from build123d import *

# Parameters (mm, degrees)
EXTRUDE1_DEPTH     = 0.65
CUT_EXTRUDE1_REACH = 20.654
SKETCH3_R          = 0.5
LPATTERN1_COUNT    = 3
LPATTERN1_PITCH    = 2.54


with BuildPart() as part:
    # Sketch1 → Extrude1 (new, symmetric)
    with BuildSketch(Plane.XY):
        Polygon((5.075, -12.4), (5.075, -5.4), (13.875, -5.4), (13.875, 5.4), (-13.875, 5.4), (-13.875, -5.4), (-5.075, -5.4), (-5.075, -12.4), align=None)
    extrude(amount=EXTRUDE1_DEPTH, both=True)

    # Sketch3 → Cut-Extrude1 (cut, up to next)
    with BuildSketch(Plane.XY.offset(0.65), mode=Mode.PRIVATE) as cut_extrude1_sk1:
        with Locations((2.54, -5.4)):
            Circle(SKETCH3_R)
    cut_extrude1_tool1 = extrude(cut_extrude1_sk1.sketch, amount=-CUT_EXTRUDE1_REACH, mode=Mode.PRIVATE) & part.part
    cut_extrude1 = cut_extrude1_tool1.solids().sort_by_distance((2.54, -5.4, 0.65))[0]
    add(cut_extrude1, mode=Mode.SUBTRACT)

    # LPattern1: Cut-Extrude1 ×3
    with Locations(*[(-i * LPATTERN1_PITCH, 0, 0) for i in range(1, LPATTERN1_COUNT)]):
        add(cut_extrude1, mode=Mode.SUBTRACT)


solid = part.part
Here's how the part is built. I have some questions about the finished solid (model axes, mm). A direction names the side the tool comes from. Coordinates: 2 decimals unless noted, no trailing zeros. Order: outer loops, then holes, each group sorted by start corner. A loop starts at its lowest first (then second) coordinate and runs counter-clockwise, first axis right, second up. Notation, with made-up numbers: (77, -31) -> (96, -31) arc R9 cw to (96, -19) -> close; hole circle Ø2 at (-11.75, -20.75). An arc over 180 degrees is marked (long way). Answer in a Markdown table with one row per item.
(1) I want a section at C-C on x = 7.75. List the corners of the cut face in (y, z) for me.
Answer key:
| item | result |
|---|---|
| outline | (-5.4, -0.65) -> (5.4, -0.65) -> (5.4, 0.65) -> (-5.4, 0.65) -> close |
(2) Thinking about a two-plate mould opening in Y: for faces 4 (the face through (0, -1, -0.65)), 5 (the face through (2.81, -4.98, 0.01)), 6 (the face through (0, -12.4, 0)), which applies, +Y half, -Y half, draft (parallel to the pull), parting line (faces both ways), or undercut?
Answer key:
| item | result |
|---|---|
| face 4 | draft |
| face 5 | undercut |
| face 6 | -Y half |
(3) Please list where these lines run through material, in increasing order: probe 1 along Y at (x, z) = (-2.54, 0); probe 2 along X at (y, z) = (-5.5, 0.3) (3 decimals); probe 3 along Y at (x, z) = (-9.75, -0.45).
Answer key:
| item | result |
|---|---|
| probe 1 | -12.4 to -5.9, -4.9 to 5.4 |
| probe 2 | -5.075 to -3.03, -2.05 to -0.49, 0.49 to 2.05, 3.03 to 5.075 |
| probe 3 | -5.4 to 5.4 |
(4) I want a section at B-B on z = 0.4. List the corners of the cut face in (x, y) for me (3 decimals).
Answer key:
| item | result |
|---|---|
| outline | (-13.875, -5.4) -> (-5.075, -5.4) -> (-5.075, -12.4) -> (5.075, -12.4) -> (5.075, -5.4) -> (13.875, -5.4) -> (13.875, 5.4) -> (-13.875, 5.4) -> close; hole circle Ø1 at (-2.54, -5.4); hole circle Ø1 at (0, -5.4); hole circle Ø1 at (2.54, -5.4) |
(5) On a 3-axis mill with a long thin cutter (end or side, diameter ignored), from which of +Z, -Z, +X, -X, +Y, -Y can I reach the whole of each face in a straight line? I mean faces 1 (the face through (0, -1, 0.65)), 2 (the face through (-5.075, -9, 0)), 3 (the face through (9, -5.4, 0)). Say none if no direction works.
Answer key:
| item | result |
|---|---|
| face 1 | +Z, +X, -X, +Y, -Y |
| face 2 | +Z, -Z, -X, -Y |
| face 3 | +Z, -Z, +X, -Y |
(6) I want a section at A-A on x = -2.54. List the corners of the cut face in (y, z) for me, then the cut area to 3 significant figures.
Answer key:
| item | result |
|---|---|
| outline | (-12.4, -0.65) -> (-5.9, -0.65) -> (-5.9, 0.65) -> (-12.4, 0.65) -> close; (-4.9, -0.65) -> (5.4, -0.65) -> (5.4, 0.65) -> (-4.9, 0.65) -> close |
| area | 21.8 mm^2 |
